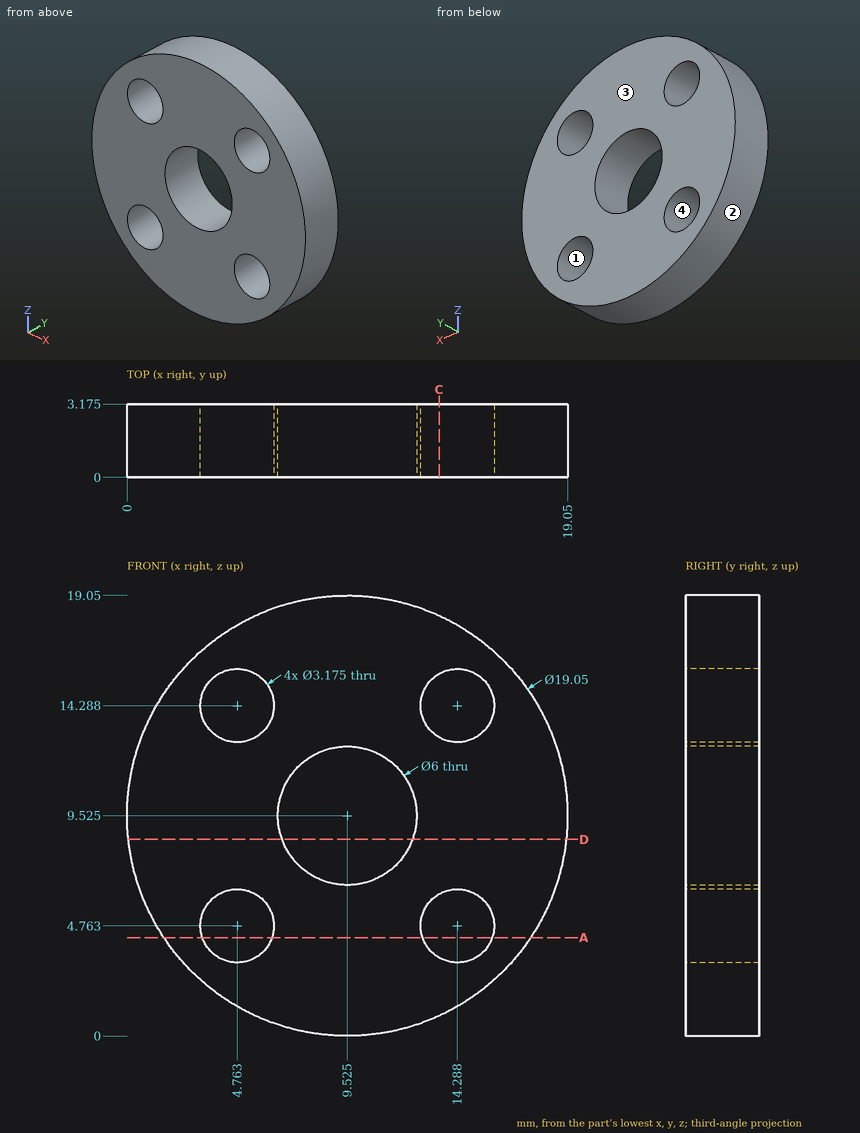
Could you check a few things on this drawing? It's one solid part, dimensions in mm from its lowest x, y, z. Round coordinates to 2 decimals unless told otherwise and drop trailing zeros. Order: outer loops, then holes, each group sorted by start corner. A loop starts at its lowest first (then second) coordinate and runs counter-clockwise, first axis right, second up. Notation, with made-up numbers: M 84,34.25 L 100,34.25 A4 cw 100,38.25 Z; hole C 79.25,73.25 d8. An arc over 180 degrees is marked long. Return JSON: item names as keys, results as strings. Group by question number.
1. I'm going to push flat-ended pins straight in: pin 1 Ø1 at (y, z) = (2.5, 11) entering from +X; pin 2 Ø1.9 at (x, z) = (14.29, 4.76) entering from +Y; pin 3 Ø1.5 at (x, y) = (15.5, 2.5) entering from -Z. Where does each tip first touch, or does it pass through?
2. If we section it at A-A on z = 4.25: List the corners of the cut face in (x, y) for me (1 decimal).
3. Please list where these lines run through material, in increasing order: probe 1 along X at (y, z) = (1.05, 13.25) (1 decimal); probe 2 along X at (y, z) = (0.5, 14.75) (1 decimal); probe 3 along Z at (x, y) = (15, 2.8) (1 decimal).
4. If we section it at C-C on x = 13.5: List the corners of the cut face in (y, z) for me (1 decimal).
5. If we mould it in two halves opening along Z, with no side actions, what happens to the marked faces 1, 2, 3 and 4? For each: pulls with the +Z half, pulls with the -Z half, needs draft (parallel to the pull), parting line crosses it, or undercut.
6. If we section it at D-D on z = 8.5: List the corners of the cut face in (x, y) for me (1 decimal).
Reply:
{
 "1": {"pin 1": "x = 19", "pin 2": "through", "pin 3": "z = 1.56"},
 "2": {"outline": "M 1.6,0 L 3.3,0 L 3.3,3.2 L 1.6,3.2 Z; M 6.3,0 L 12.8,0 L 12.8,3.2 L 6.3,3.2 Z; M 15.8,0 L 17.5,0 L 17.5,3.2 L 15.8,3.2 Z"},
 "3": {"probe 1": "0.8 to 3.6, 6 to 13.1, 15.5 to 18.3", "probe 2": "1.6 to 3.2, 6.3 to 12.8, 15.8 to 17.5", "probe 3": "1.7 to 3.3, 6.2 to 12.9, 15.7 to 17.3"},
 "4": {"outline": "M 0,0.9 L 3.2,0.9 L 3.2,3.4 L 0,3.4 Z; M 0,6.1 L 3.2,6.1 L 3.2,12.9 L 0,12.9 Z; M 0,15.7 L 3.2,15.7 L 3.2,18.2 L 0,18.2 Z"},
 "5": {"face 1": "undercut", "face 2": "parting line crosses it", "face 3": "needs draft", "face 4": "undercut"},
 "6": {"outline": "M 0.1,0 L 6.7,0 L 6.7,3.2 L 0.1,3.2 Z; M 12.3,0 L 19,0 L 19,3.2 L 12.3,3.2 Z"}
}
